Input: part model. Units: mm. Frame: model coordinates. A direction names the side the tool comes from. Round coordinates to 2 decimals unless told otherwise and drop trailing zeros. Loops run counter-clockwise (first coordinate to the right, second up) from the corner with the lowest first, then second, coordinate; pieces in that order, holes last. Notation, with made-up numbers: (0, 52.5) -> (10, 52.5) arc R22 cw to (10, 77.5) -> close; hole circle Ø2 at (58.25, 42). An arc over 180 degrees is marked (long way). Answer in a Markdown table with one row per item. Add a question column.
Q1. Reachability of faces 1 (the face through (-7.6, -22, 4)), 2 (the face through (-2.49, 28.75, -6.38)), 3 (the face through (0, -6.11, -8.13)) from +Z, -Z, +X, -X, +Y, -Y: full face, straight path, thin tool, end or side. Return the list, or none.
Q2. Section C-C, the plane x = -4.5. Output: boundary loops of the cut face in (y, z).
Q3. Pin query (flat end, axial travel): pin 1 (4 mm diameter, centred on x = 0.5, y = 18, fed in from -Z); pin 2 (4 mm diameter, centred on y = 14.5, z = -11, fed in from +X); pin 3 (3 mm diameter, centred on x = -6.5, y = -19.5, fed in from +Z). Return the tip coordinate at first contact, or that it passes through.
Q4. Mould query, pull axis Z, two halves, no side actions, for faces 4 (the face through (-2.61, -30.09, -3.95)), 5 (the face through (0.9, -6.11, 8.13)), 6 (the face through (-6.7, -22, -4)), 7 (the face through (1.5, -25, 16)). Classes: pulls with the +Z half, pulls with the -Z half, needs draft (parallel to the pull), parting line crosses it, or undercut.
Q5. Ray query, L1, parallel to Y at x = 0.5, z = 6.5; L2, parallel to Y at x = -6, z = 15; L3, parallel to Z at x = -4.75, y = 16.5. Return the intervals inside material, ascending. Write a range as from..to.
```python
from build123d import *


with BuildPart() as part:
    # Croquis1 → Revolución1 (revolve)
    with BuildSketch(Plane.XY, mode=Mode.PRIVATE) as revoluci_n1_sk:
        with BuildLine():
            Line((0.9, -10), (0.9, -13.606089524))
            ThreePointArc((0.9, -13.606089524), (0.830417568, -13.972590751), (0.631353702, -14.288087884))
            Line((0.631353702, -14.288087884), (-6.67313537, -22.121193408))
            ThreePointArc((-6.67313537, -22.121193408), (-6.693041757, -22.152743121), (-6.7, -22.189393244))
            Line((-6.7, -22.189393244), (-6.7, -29.35))
            ThreePointArc((-6.7, -29.35), (-6.670710678, -29.420710678), (-6.6, -29.45))
            Line((-6.6, -29.45), (1.5, -29.45))
            Line((1.5, -29.45), (1.5, -30.35))
            Line((1.5, -30.35), (-6.6, -30.35))
            ThreePointArc((-6.6, -30.35), (-7.307106781, -30.057106781), (-7.6, -29.35))
            Line((-7.6, -29.35), (-7.6, -22.189393244))
            ThreePointArc((-7.6, -22.189393244), (-7.530417568, -21.822892017), (-7.331353702, -21.507394884))
            Line((-7.331353702, -21.507394884), (-0.02686463, -13.67428936))
            ThreePointArc((-0.02686463, -13.67428936), (-0.006958243, -13.642739647), (0, -13.606089524))
            Line((0, -13.606089524), (0, -10))
            Line((0, -10), (0.9, -10))
        make_face()
    revolve(revoluci_n1_sk.sketch.rotate(Axis((0, 0, 0), (1, 0, 0)), 270), axis=Axis((0, 0, 0), (1, 0, 0)))


solid = part.part
```
Answer block:
| question | item | result |
|---|---|---|
| 1 | face 1 | +Z, -Z, -X, +Y, -Y |
| 1 | face 2 | +X |
| 1 | face 3 | -X |
| 2 | outline | circle Ø60.7 at (0, 0); circle Ø39.58 at (0, 0); hole circle Ø58.9 at (0, 0); hole circle Ø36.94 at (0, 0) |
| 3 | pin 1 | z = -25.79 |
| 3 | pin 2 | x = -1.15 |
| 3 | pin 3 | z = 24.44 |
| 4 | face 4 | parting line crosses it |
| 4 | face 5 | undercut |
| 4 | face 6 | undercut |
| 4 | face 7 | needs draft |
| 5 | L1 | -29.65..-28.72, -12.88..-7.6, 7.6..12.88, 28.72..29.65 |
| 5 | L2 | -26.38..-25.34, -15.26..-13.35, 13.35..15.26, 25.34..26.38 |
| 5 | L3 | -25.47..-24.39, -11.41..-8.88, 8.88..11.41, 24.39..25.47 |
